Can you work these out from the drawing? Everything is in mm from the part's minimum corner. A direction names the side the tool comes from. Coordinates: 2 decimals unless noted, no trailing zeros. Write each loop counter-clockwise with the first axis right and the second up, starting at its lowest first coordinate (ties: lowest second). Pieces come first, ordered by that corner, then holes.
(1) Thinking about a two-plate mould opening in Z: for the marked faces 5, 6, 7 and 8, which applies, released by +Z, released by -Z, zero draft, split by the parting line, or undercut?
(2) Please list where these lines run through material, in increasing order: probe 1 along Y at (x, z) = (20, 34); probe 2 along X at (y, z) = (46.5, 20); probe 3 along Z at (x, y) = (26, 38.5).
(3) For pin 1 Ø6 at (y, z) = (16.5, 9.5) entering from +X; pin 2 Ø10 at (x, z) = (42.5, 8.5) entering from -Y; pin 3 Ø12 at (x, z) = (67.5, 30.5) entering from -Y, each with a flat end and sliding along its axis, tell me the tip position at first contact or that it passes through.
(4) Imagine slicing it at D-D, the plane y = 53.5. List the corners of the cut face in (x, z) for me.
(5) Imagine slicing it at A-A, the plane y = 10.5. List the corners of the cut face in (x, z) for me.
(6) Which directions (+Z, -Z, +X, -X, +Y, -Y) give clear straight access to the entire face, cutting with the end or side of a thin tool? Please do the marked faces 1, 2, 3 and 4.
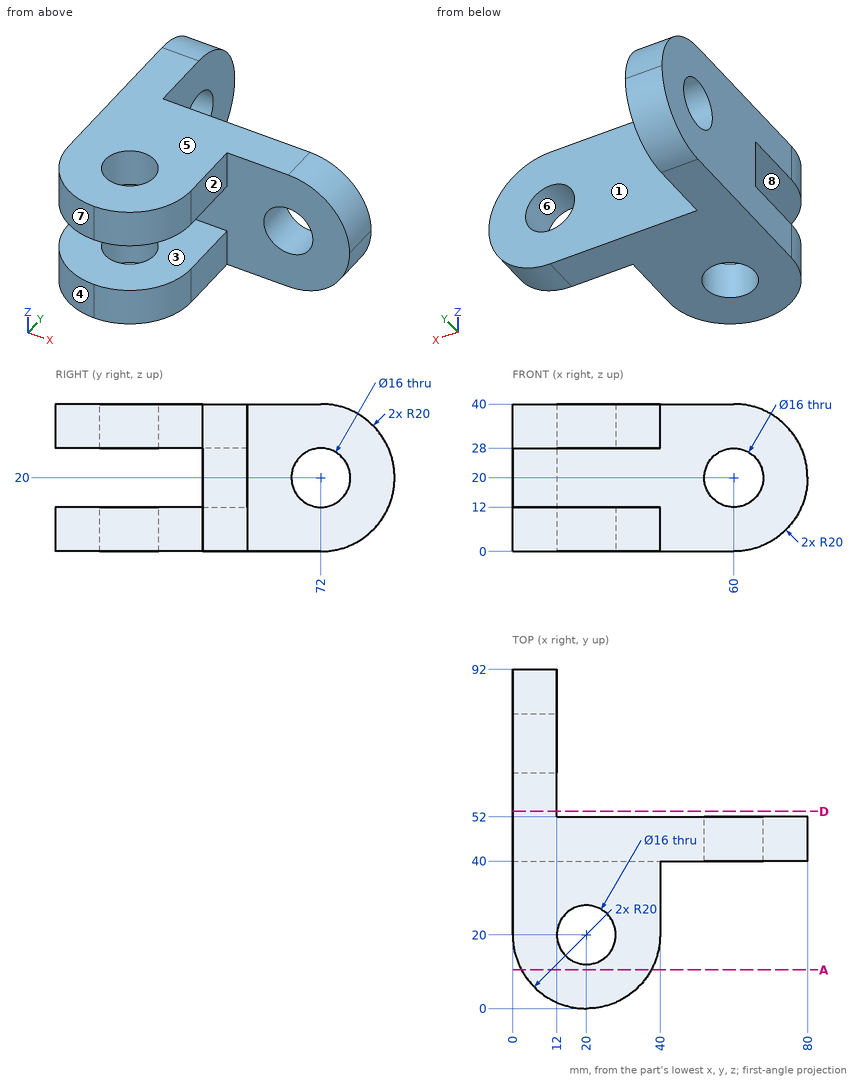
Recorded:
1. face 5: released by +Z
1. face 6: undercut
1. face 7: zero draft
1. face 8: undercut
2. probe 1: y = 0 to 12, 28 to 52
2. probe 2: x = 0 to 52, 68 to 80
2. probe 3: z = 0 to 12, 28 to 40
3. pin 1: stops at x = 39.99
3. pin 2: stops at y = 10.32
3. pin 3: stops at y = 40
4. outline: (0, 0) - (12, 0) - (12, 40) - (0, 40) - close
5. outline: (2.4, 0) - (37.6, 0) - (37.6, 12) - (2.4, 12) - close; (2.4, 28) - (37.6, 28) - (37.6, 40) - (2.4, 40) - close
6. face 1: +Z, -Z, +X, +Y
6. face 2: +Z, -Z, +X, -Y
6. face 3: +X, -X, -Y
6. face 4: +Z, -Z, -X, -Y
